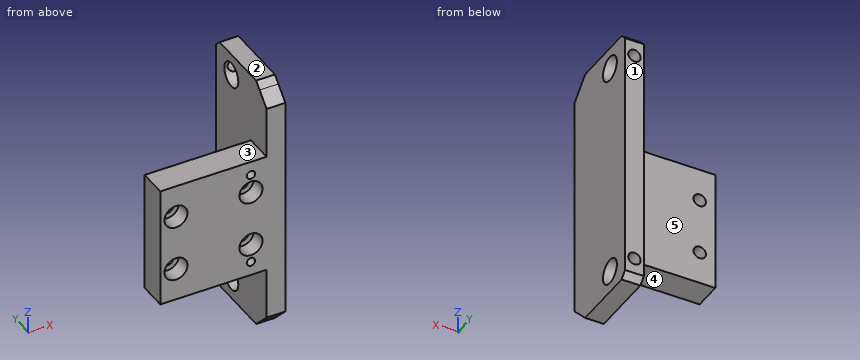
from build123d import *

# Parameters (mm, degrees)
SKETCH1_W           = 34
SKETCH1_H           = 39
SKETCH1_R           = 2
BOSS_EXTRUDE1_DEPTH = 5
SKETCH2_W           = 6
SKETCH2_H           = 84
BOSS_EXTRUDE2_DEPTH = 25
CUT_EXTRUDE2_REACH  = 65.159
SKETCH3_R           = 4
CHAMFER1_SIZE       = 2
SKETCH4_R           = 2
CUT_EXTRUDE3_DEPTH  = 10
BOSS_EXTRUDE3_DEPTH = 4
SKETCH6_R           = 3.7
CUT_EXTRUDE4_DEPTH  = 5
CHAMFER2_SIZE       = 4
CUT_EXTRUDE5_REACH  = 57.982
SKETCH7_R           = 1.35


with BuildPart() as part:
    # Sketch1 → Boss-Extrude1 (new body)
    with BuildSketch(Plane(origin=(0, 0, 0), x_dir=(1, 0, 0), z_dir=(0, 1, 0))):
        Rectangle(SKETCH1_W, SKETCH1_H)
        with Locations(Location((-12, -9, 0), (0, 0, 270))):
            Circle(SKETCH1_R, mode=Mode.SUBTRACT)
        with Locations(Location((12, -9, 0), (0, 0, 90))):
            Circle(SKETCH1_R, mode=Mode.SUBTRACT)
        with Locations(Location((12, 9, 0), (0, 0, 270))):
            Circle(SKETCH1_R, mode=Mode.SUBTRACT)
        with Locations(Location((-12, 9, 0), (0, 0, 90))):
            Circle(SKETCH1_R, mode=Mode.SUBTRACT)
    extrude(amount=BOSS_EXTRUDE1_DEPTH)

    # Sketch2 → Boss-Extrude2 (add)
    with BuildSketch(Plane.XZ):
        with Locations((20, 0)):
            Rectangle(SKETCH2_W, SKETCH2_H)
    extrude(amount=-BOSS_EXTRUDE2_DEPTH)

    # Sketch3 → Cut-Extrude2 (cut, up to next)
    with BuildSketch(Plane(origin=(23, 0, 0), x_dir=(0, 0, -1), z_dir=(1, 0, 0)), mode=Mode.PRIVATE) as cut_extrude2_sk1:
        with Locations((-35, 16.275206728)):
            Circle(SKETCH3_R)
    cut_extrude2_tool1 = extrude(cut_extrude2_sk1.sketch, amount=-CUT_EXTRUDE2_REACH, mode=Mode.PRIVATE) & part.part
    # Sketch3 → Cut-Extrude2 (cut, up to next)
    with BuildSketch(Plane(origin=(23, 0, 0), x_dir=(0, 0, -1), z_dir=(1, 0, 0)), mode=Mode.PRIVATE) as cut_extrude2_sk2:
        with Locations((35, 16.275206728)):
            Circle(SKETCH3_R)
    cut_extrude2_tool2 = extrude(cut_extrude2_sk2.sketch, amount=-CUT_EXTRUDE2_REACH, mode=Mode.PRIVATE) & part.part
    add(cut_extrude2_tool1.solids().sort_by_distance((23, 16.275207, 35))[0], mode=Mode.SUBTRACT)
    add(cut_extrude2_tool2.solids().sort_by_distance((23, 16.275207, -35))[0], mode=Mode.SUBTRACT)

    # Chamfer1
    chamfer1_edges = [part.edges().sort_by_distance(p)[0] for p in [
        (20, 25, -42),
        (20, 25, 42),
        (20, 0, 42),
        (20, 0, -42),
    ]]
    chamfer(chamfer1_edges, length=CHAMFER1_SIZE)

    # Sketch4 → Cut-Extrude3 (cut)
    with BuildSketch(Plane(origin=(0, 25, 0), x_dir=(1, 0, 0), z_dir=(0, 1, 0))):
        with Locations(Location((20, 35, 0), (0, 0, 270))):
            Circle(SKETCH4_R)
        with Locations(Location((20, -35, 0), (0, 0, 270))):
            Circle(SKETCH4_R)
    extrude(amount=-CUT_EXTRUDE3_DEPTH, mode=Mode.SUBTRACT)

    # Sketch5 → Boss-Extrude3 (add)
    with BuildSketch(Plane.XZ):
        Polygon((17, -19.5), (17, -40), (23, -40), (23, 40), (17, 40), (17, 19.5), (-17, 19.5), (-17, -19.5), align=None)
    extrude(amount=BOSS_EXTRUDE3_DEPTH)

    # Sketch6 → Cut-Extrude4 (cut)
    with BuildSketch(Plane.XZ.offset(4)):
        with Locations(Location((-12, -9, 0), (0, 0, 270))):
            Circle(SKETCH6_R)
        with Locations(Location((12, -9, 0), (0, 0, 90))):
            Circle(SKETCH6_R)
        with Locations(Location((12, 9, 0), (0, 0, 270))):
            Circle(SKETCH6_R)
        with Locations(Location((-12, 9, 0), (0, 0, 90))):
            Circle(SKETCH6_R)
    extrude(amount=-CUT_EXTRUDE4_DEPTH, mode=Mode.SUBTRACT)

    # Chamfer2
    chamfer2_edges = [part.edges().sort_by_distance(p)[0] for p in [
        (20, -4, 40),
        (20, -4, -40),
    ]]
    chamfer(chamfer2_edges, length=CHAMFER2_SIZE - 0.0001)  # a hair under: the kernel refuses the full size

    # Sketch7 → Cut-Extrude5 (cut, up to next)
    with BuildSketch(Plane.XZ.offset(4), mode=Mode.PRIVATE) as cut_extrude5_sk1:
        with Locations(Location((12, 15, 0), (0, 0, 270))):
            Circle(SKETCH7_R)
    cut_extrude5_tool1 = extrude(cut_extrude5_sk1.sketch, amount=-CUT_EXTRUDE5_REACH, mode=Mode.PRIVATE) & part.part
    # Sketch7 → Cut-Extrude5 (cut, up to next)
    with BuildSketch(Plane.XZ.offset(4), mode=Mode.PRIVATE) as cut_extrude5_sk2:
        with Locations(Location((12, -15, 0), (0, 0, 270))):
            Circle(SKETCH7_R)
    cut_extrude5_tool2 = extrude(cut_extrude5_sk2.sketch, amount=-CUT_EXTRUDE5_REACH, mode=Mode.PRIVATE) & part.part
    add(cut_extrude5_tool1.solids().sort_by_distance((12, -4, 15))[0], mode=Mode.SUBTRACT)
    add(cut_extrude5_tool2.solids().sort_by_distance((12, -4, -15))[0], mode=Mode.SUBTRACT)


solid = part.part
Source: CAD feature listing. Evaluate the final solid. Frame: model axes, mm. Face numbers are marked on the shaded views. A direction names the side the tool comes from. Round coordinates to 2 decimals unless told otherwise and drop trailing zeros. Loops run counter-clockwise (first coordinate to the right, second up) from the corner with the lowest first, then second, coordinate; pieces in that order, holes last. Notation, with made-up numbers: (8.25, -34) - (37.25, -34) arc R21 cw to (37.25, 2) - close; hole circle Ø3 at (22, 38.5). An arc over 180 degrees is marked (long way). Write item = value, one per line. Start each with the question number.
Item 1: Section query A-A on z = 15. Output: boundary loops of the cut face in (x, y).
Item 2: Reachability of the marked faces 1, 2, 3, 4 and 5 from +Z, -Z, +X, -X, +Y, -Y: full face, straight path, thin tool, end or side. Return the list, or none.
Item 3: First-contact query: pin 1 Ø10 at (x, y) = (1.5, -0.5) entering from +Z; pin 2 Ø6 at (x, z) = (-12, -9) entering from -Y; pin 3 Ø7 at (x, y) = (1.5, 1) entering from -Z. Flat tips, straight axial feed; report the tip coordinate or a pass-through.
Item 4: Section query C-C on y = 17.5. Output: boundary loops of the cut face in (x, z).
Item 5: Section query B-B on x = -12. Output: boundary loops of the cut face in (y, z).
Item 6: Material intervals for line 1 (X direction, y = 2.65, z = 9); line 2 (Z direction, x = -12, y = 2.8); line 3 (X direction, y = -2.6, z = 9), sorted ascending.
Item 7: Section query D-D on z = -9. Output: boundary loops of the cut face in (x, y).
Results list:
q1.outline = (-17, -4) - (10.65, -4) - (10.65, 5) - (-17, 5) - close; (13.35, -4) - (23, -4) - (23, 25) - (17, 25) - (17, 5) - (13.35, 5) - close
q2.face_1 = +Z, -Z, +X, -X, +Y
q2.face_2 = +Z, +X, -X, +Y, -Y
q2.face_3 = +Z, -X, +Y, -Y
q2.face_4 = -Z, -X, +Y, -Y
q2.face_5 = +Z, -Z, -X, +Y
q3.pin_1 = 19.5
q3.pin_2 = 1
q3.pin_3 = -19.5
q4.outline = (17, -42) - (23, -42) - (23, -38.81) - (17, -38.81) - close; (17, -31.19) - (23, -31.19) - (23, 31.19) - (17, 31.19) - close; (17, 38.81) - (23, 38.81) - (23, 42) - (17, 42) - close
q5.outline = (-4, -19.5) - (5, -19.5) - (5, -11) - (1, -11) - (1, -12.7) - (-4, -12.7) - close; (-4, -5.3) - (1, -5.3) - (1, -7) - (5, -7) - (5, 7) - (1, 7) - (1, 5.3) - (-4, 5.3) - close; (-4, 12.7) - (1, 12.7) - (1, 11) - (5, 11) - (5, 19.5) - (-4, 19.5) - close
q6.line_1 = -17 to -14, -10 to 10, 14 to 23
q6.line_2 = -19.5 to -11, -7 to 7, 11 to 19.5
q6.line_3 = -17 to -15.7, -8.3 to 8.3, 15.7 to 23
q7.outline = (-17, -4) - (-15.7, -4) - (-15.7, 1) - (-14, 1) - (-14, 5) - (-17, 5) - close; (-10, 1) - (-8.3, 1) - (-8.3, -4) - (8.3, -4) - (8.3, 1) - (10, 1) - (10, 5) - (-10, 5) - close; (14, 1) - (15.7, 1) - (15.7, -4) - (23, -4) - (23, 25) - (17, 25) - (17, 5) - (14, 5) - close
